The model under review builds one solid part; all positions refer to its coordinate system, in mm. A direction names the side the tool comes from. Coordinates: 2 decimals unless noted, no trailing zeros. Write each loop counter-clockwise with the first axis right and the second up, starting at its lowest first coordinate (ties: lowest second). Pieces come first, ordered by that corner, then holes. Notation, with made-up numbers: (39.25, 24) - (83.25, 24) arc R25 ccw to (83.25, 63) - close; hole circle Ø1 at (5.25, 86.25). An arc over 180 degrees is marked (long way). Return JSON: item names as keys, results as strings. Group by question number.
(1) For pin 1 Ø3 at (x, y) = (20.5, 55) entering from +Z; pin 2 Ø6 at (x, z) = (41, -2.5) entering from +Y; pin 3 Ø19.5 at (y, z) = (90, -25) entering from -X, all flat-tipped, find the tip position at first contact; note any pin that passes through.
(2) Draft analysis for pull direction Z (two halves, no side actions). For faces 1 (the face through (-1, 48, 0)), 2 (the face through (-1.627, 76.606, 7.395)), 3 (the face through (-42.83, 4.93, -22.737)), 4 (the face through (-1, 48, -39.3)), state which applies: released by +Z, released by -Z, zero draft, split by the parting line, or undercut.
(3) We need section B-B on z = -19.65. State the section outline as (x, y) points.
(4) Tool access review of faces 5 (the face through (0, 89, 15)), 6 (the face through (-9.184, 117.288, -19.375)), 7 (the face through (20, 65, -19)), 8 (the face through (-20, 65, -19)), 9 (the face through (37.17, 4.93, -22.737)): name each direction out of +Z, -Z, +X, -X, +Y, -Y from which nothing blocks a thin tool from reaching the whole face with its end or side.
(5) To check wall thickness, follow L1, parallel to X at y = 5, z = -19.65; L2, parallel to Z at x = 40, y = 6.5; L3, parallel to X at y = 4, z = -19. State the ranges of each line that lie inside material, in increasing order. Write a range as from..to.
(6) We need section D-D on y = 49.5. State the section outline as (x, z) points, then the cut area to 3 significant figures.
(7) We need section C-C on z = -35. State the section outline as (x, y) points.
(8) We need section A-A on x = -40. State the section outline as (y, z) points, then the cut area to 3 significant figures.
Autodesk Inventor part; units mm, degrees
ref_plane "YZ Plane" through (0, 0, 0) normal (1, 0, 0) x (0, 1, 0)
ref_plane "XZ Plane" through (0, 0, 0) normal (0, 1, 0) x (-1, 0, 0)
ref_plane "XY Plane" through (0, 0, 0) normal (0, 0, 1) x (1, 0, 0)
sketch "Sketch3" plane through (0, 0, 0) normal (0, 0, 1) x (1, 0, 0)
  line L0 (0, 0) -> (60, 0)
  line L1 (60, 0) -> (60, 10)
  line L2 (60, 10) -> (20, 10)
  line L3 (20, 10) -> (20, 120.986)
  line L4 (0, 0) -> (0, 29.8306) construction
  line L5 (0, 0) -> (-60, 0)
  line L6 (-60, 0) -> (-60, 10)
  line L7 (-60, 10) -> (-20, 10)
  line L8 (-20, 10) -> (-20, 120.986)
  line L9 (799.716, 113.486) -> (799.716, 376.2074) construction
  line L10 (0, 113.486) -> (18.1144, 120.986)
  line L11 (18.1144, 120.986) -> (20, 120.986)
  line L12 (-18.1144, 120.986) -> (0, 113.486)
  line L13 (-20, 120.986) -> (-18.1144, 120.986)
  dimension "d10" = 60
  dimension "d11" = 10
  dimension "d41" = 18.1144
  dimension "d44" = 110.986
  dimension "d45" = 7.5
  dimension "d46" = 40
  dimension "d47" = 110.986
extrude "Extrusion1" add sketch "Sketch3" against normal blind 39.3
sketch "Sketch4" plane through (0, 0, 0) normal (0, 0, 1) x (1, 0, 0)
  circle A0 centre (0, 89) radius 12.5
  point P0 (0, 0)
  dimension "d20" = 25
extrude "Extrusion2" add sketch "Sketch4" along normal blind 15
fillet "Fillet1" radius 2 4 edges at (60, 5, 0) (60, 5, -39.3) (-60, 5, 0) (-60, 5, -39.3)
sketch "Sketch5" plane through (-20, 10, 0) normal (0, 1, 0) x (1, 0, 0)
  line L0 (-38, 39.3) -> (0, 39.3)
  line L1 (40, 39.3) -> (78, 39.3)
  line L2 (-40, 2) -> (-40, 37.3)
  line L3 (80, 2) -> (80, 37.3)
  point P0 (20, 0)
  point P1 (-20, 19.65)
  point P2 (60, 19.65)
  dimension "d24" = 19.65
  dimension "d25" = 19.65
  dimension "d26" = 20
  dimension "d27" = 20
hole "Hole1" at (-40, 10, -19.65) at (40, 10, -19.65) direction (0, -1, 0) diameter 8.376 end through all
equation "\"d47\" = d44"
properties part number "Stop sliding"
Ans:
{
 "1": {"pin 1": "z = 0", "pin 2": "y = 10", "pin 3": "x = -20"},
 "2": {"face 1": "released by +Z", "face 2": "zero draft", "face 3": "undercut", "face 4": "released by -Z"},
 "3": {"outline": "(-60, 0) - (-44.19, 0) - (-44.19, 10) - (-60, 10) - close; (-35.81, 0) - (35.81, 0) - (35.81, 10) - (20, 10) - (20, 120.99) - (18.11, 120.99) - (0, 113.49) - (-18.11, 120.99) - (-20, 120.99) - (-20, 10) - (-35.81, 10) - close; (44.19, 0) - (60, 0) - (60, 10) - (44.19, 10) - close"},
 "4": {"face 5": "+Z, +X, -X, +Y, -Y", "face 6": "+Z, -Z, +Y", "face 7": "+Z, -Z, +X, +Y", "face 8": "+Z, -Z, -X, +Y", "face 9": "+Y, -Y"},
 "5": {"L1": "-60..-44.19, -35.81..35.81, 44.19..60", "L2": "-39.3..-23.84, -15.46..0", "L3": "-60..-44.14, -35.86..35.86, 44.14..60"},
 "6": {"outline": "(-20, -39.3) - (20, -39.3) - (20, 0) - (-20, 0) - close", "area": "1,570 mm²"},
 "7": {"outline": "(-60, 0) - (60, 0) - (60, 10) - (20, 10) - (20, 120.99) - (18.11, 120.99) - (0, 113.49) - (-18.11, 120.99) - (-20, 120.99) - (-20, 10) - (-60, 10) - close"},
 "8": {"outline": "(0, -39.3) - (10, -39.3) - (10, -23.84) - (0, -23.84) - close; (0, -15.46) - (10, -15.46) - (10, 0) - (0, 0) - close", "area": "309 mm²"}
}
